Work out the finished part from the listing and answer in its coordinate system (mm). A direction names the side the tool comes from. Round coordinates to 2 decimals unless told otherwise and drop trailing zeros. Order: outer loops, then holes, each group sorted by start corner. A loop starts at its lowest first (then second) coordinate and runs counter-clockwise, first axis right, second up. Notation, with made-up numbers: (40.25, 49.5) - (71.25, 49.5) arc R31 cw to (71.25, 84.5) - close; hole circle Ø1 at (74, -22). An arc over 180 degrees is marked (long way). Answer in a Markdown table with one row per item.
from build123d import *

# Parameters (mm, degrees)
SKETCH1_W                 = 279.4
SKETCH1_H                 = 364
BOSS_EXTRUDE1_DEPTH       = 10
SKETCH2_W                 = 101.6
SKETCH2_H                 = 101.6
CUT_EXTRUDE1_DEPTH        = 230.652106457
LPATTERN1_COUNT           = 2
LPATTERN1_PITCH           = 110.265
LPATTERN2_COUNT           = 2
LPATTERN2_PITCH           = 110.265
LPATTERN3_COUNT           = 2
LPATTERN3_PITCH           = 114.82
LPATTERN3_COPY_1_SKETCH_W = 101.6
LPATTERN3_COPY_1_SKETCH_H = 101.6
LPATTERN3_COPY_1_DEPTH    = 230.652106457
LPATTERN3_COPY_2_SKETCH_W = 101.6
LPATTERN3_COPY_2_SKETCH_H = 101.6
LPATTERN3_COPY_2_DEPTH    = 230.652106457
SKETCH3_W                 = 313.16
SKETCH3_H                 = 10
BOSS_EXTRUDE2_DEPTH       = 25.4
SKETCH4_R                 = 3.5687
CUT_EXTRUDE2_DEPTH        = 10


with BuildPart() as part:
    # Sketch1 → Boss-Extrude1 (new body)
    with BuildSketch(Plane(origin=(0, 0, 0), x_dir=(1, 0, 0), z_dir=(0, 1, 0))):
        Rectangle(SKETCH1_W, SKETCH1_H)
    extrude(amount=BOSS_EXTRUDE1_DEPTH)

    # Sketch2 → Cut-Extrude1 (cut, through all)
    with BuildSketch(Plane(origin=(0, 10, 0), x_dir=(1, 0, 0), z_dir=(0, 1, 0))):
        with Locations((-63.5, 0)):
            Rectangle(SKETCH2_W, SKETCH2_H)
    cut_extrude1 = extrude(amount=-CUT_EXTRUDE1_DEPTH, mode=Mode.SUBTRACT)

    # LPattern1: Cut-Extrude1 ×2
    with Locations(*[(0, 0, -i * LPATTERN1_PITCH) for i in range(1, LPATTERN1_COUNT)]):
        add(cut_extrude1, mode=Mode.SUBTRACT)

    # LPattern2: Cut-Extrude1 ×2
    with Locations(*[(0, 0, i * LPATTERN2_PITCH) for i in range(1, LPATTERN2_COUNT)]):
        add(cut_extrude1, mode=Mode.SUBTRACT)

    # LPattern3: Cut-Extrude1 ×2
    with Locations(*[(i * LPATTERN3_PITCH, 0, 0) for i in range(1, LPATTERN3_COUNT)]):
        add(cut_extrude1, mode=Mode.SUBTRACT)

    # LPattern3 copy 1 sketch → LPattern3 copy 1 (cut, through all)
    with BuildSketch(Plane(origin=(114.82, 10, -110.265), x_dir=(1, 0, 0), z_dir=(0, 1, 0))):
        with Locations((-63.5, 0)):
            Rectangle(LPATTERN3_COPY_1_SKETCH_W, LPATTERN3_COPY_1_SKETCH_H)
    extrude(amount=-LPATTERN3_COPY_1_DEPTH, mode=Mode.SUBTRACT)

    # LPattern3 copy 2 sketch → LPattern3 copy 2 (cut, through all)
    with BuildSketch(Plane(origin=(114.82, 10, 110.265), x_dir=(1, 0, 0), z_dir=(0, 1, 0))):
        with Locations((-63.5, 0)):
            Rectangle(LPATTERN3_COPY_2_SKETCH_W, LPATTERN3_COPY_2_SKETCH_H)
    extrude(amount=-LPATTERN3_COPY_2_DEPTH, mode=Mode.SUBTRACT)

    # Sketch3 → Boss-Extrude2 (add)
    with BuildSketch(Plane.ZY.offset(139.7)):
        with Locations((0, 5)):
            Rectangle(SKETCH3_W, SKETCH3_H)
    extrude(amount=BOSS_EXTRUDE2_DEPTH)

    # Sketch4 → Cut-Extrude2 (cut)
    with BuildSketch(Plane.XZ):
        with Locations(Location((127.00134615, -118.505273154, 0), (0, 0, 270))):
            Circle(SKETCH4_R)
        with Locations(Location((127.00134615, -143.905273154, 0), (0, 0, 270))):
            Circle(SKETCH4_R)
        with Locations(Location((-152.4, -118.505273154, 0), (0, 0, 270))):
            Circle(SKETCH4_R)
        with Locations(Location((-152.4, -143.905273154, 0), (0, 0, 270))):
            Circle(SKETCH4_R)
    cut_extrude2 = extrude(amount=-CUT_EXTRUDE2_DEPTH, mode=Mode.SUBTRACT)

    # Mirror1: Cut-Extrude2 across plane
    add(cut_extrude2.mirror(Plane.XY), mode=Mode.SUBTRACT)


solid = part.part
1) This flat-tipped pin is pushed along its axis until it touches: pin 1 (4.5 mm diameter, centred on x = 127, z = -143.91, fed in from +Y). Where does it stop, or does it pass through?
Filled in:
| item | result |
|---|---|
| pin 1 | passes through |
2) Find section A-A, the plane x = 57.5. Give the vertices of the cut face in (y, z) (3 decimals), then the cut area to 3 significant figures.
Filled in:
| item | result |
|---|---|
| outline | (0, -182) - (10, -182) - (10, -161.065) - (0, -161.065) - close; (0, -59.465) - (10, -59.465) - (10, -50.8) - (0, -50.8) - close; (0, 50.8) - (10, 50.8) - (10, 59.465) - (0, 59.465) - close; (0, 161.065) - (10, 161.065) - (10, 182) - (0, 182) - close |
| area | 592 mm^2 |
3) The mould has two halves that part along Z. Classify faces 4 (the face through (-2, 5, 182)), 5 (the face through (-152, 5, -156.58)), 6 (the face through (-114.3, 5, 1)): released by +Z, released by -Z, zero draft, split by the parting line, or undercut.
Filled in:
| item | result |
|---|---|
| face 4 | released by +Z |
| face 5 | released by -Z |
| face 6 | undercut |
4) Which of the six approach directions +Z, -Z, +X, -X, +Y, -Y give full straight-line access (tool end or side, diameter ignored) to faces 1 (the face through (-152, 5, 156.58)), 2 (the face through (51, 5, 161.065)), 3 (the face through (139.7, 5, 3))?
Filled in:
| item | result |
|---|---|
| face 1 | +Z, -X, +Y, -Y |
| face 2 | +Y, -Y |
| face 3 | +Z, -Z, +X, +Y, -Y |
5) Find section C-C, the plane y = 5. Give the number of separate pieces and of enclosed holes in the cut face, then the cut area to 3 significant figures.
Filled in:
| item | result |
|---|---|
| separate pieces | 1 |
| enclosed holes | 14 |
| area | 47,400 mm^2 |
6) Find the intervals of material crossed by probe 1 along Z at (x, y) = (-58, 6) (3 decimals); probe 2 along X at (y, z) = (7, -151); probe 3 along X at (y, z) = (1, 163), in increasing order. Write a range as from..to.
Filled in:
| item | result |
|---|---|
| probe 1 | z = -182..-161.065, -59.465..-50.8, 50.8..59.465, 161.065..182 |
| probe 2 | x = -165.1..-114.3, -12.7..0.52, 102.12..139.7 |
| probe 3 | x = -139.7..139.7 |
7) Find section B-B, the plane z = 70.5. Give the vertices of the cut face in (x, y).
Filled in:
| item | result |
|---|---|
| outline | (-165.1, 0) - (-114.3, 0) - (-114.3, 10) - (-165.1, 10) - close; (-12.7, 0) - (0.52, 0) - (0.52, 10) - (-12.7, 10) - close; (102.12, 0) - (139.7, 0) - (139.7, 10) - (102.12, 10) - close |
